The listing builds one solid part. Answer for the finished solid, in the listing's coordinates (mm). Round coordinates to 2 decimals unless told otherwise and drop trailing zeros. Order: outer loops, then holes, each group sorted by start corner. A loop starts at its lowest first (then second) coordinate and runs counter-clockwise, first axis right, second up. Notation, with made-up numbers: (-13, 54.5) -> (27, 54.5) arc R20 ccw to (27, 71.5) -> close; hole circle Ø10 at (50.5, -19). An arc over 180 degrees is marked (long way). Answer in a Markdown table with one row per item. Add a question column.
```python
from build123d import *

# Parameters (mm, degrees)
F3_START      = 698.5
F2_W          = 2438.4
F2_H          = 457.2
F2_R          = 38.1
F3_DEPTH      = 38.1
F4_DEPTH      = 736.6
F5_R          = 38.1
F6_DEPTH      = 228.6
F6_DEPTH_BACK = 228.6
F7_R          = 25.4
F8_SIZE       = 2.54


# Not quite as in the source:
# - a variable given as a bare number and used for a length is read in inches; the dataset says mm whatever the document's units were


with BuildPart() as f3:
    # F2 (on Top) → F3 (new body)
    with BuildSketch(Plane.XY.offset(F3_START)):
        Rectangle(F2_W, F2_H)
        with Locations((-914.4, 0)):
            Circle(F2_R, mode=Mode.SUBTRACT)
        with Locations((914.4, 0)):
            Circle(F2_R, mode=Mode.SUBTRACT)
        with Locations((-914.4, 0)):
            Circle(F2_R)
        with Locations((914.4, 0)):
            Circle(F2_R)
    extrude(amount=F3_DEPTH)

    # F2 (on Top) → F4 (join)
    with BuildSketch(Plane.XY):
        with Locations((-914.4, 0)):
            Circle(F2_R)
        with Locations((914.4, 0)):
            Circle(F2_R)
    extrude(amount=F4_DEPTH)

    # F5 (on Front) → F6 (join, two sides)
    with BuildSketch(Plane.XZ) as f6_sk:
        with Locations((-914.4, 0)):
            Circle(F5_R)
        with Locations((914.4, 0)):
            Circle(F5_R)
    extrude(amount=F6_DEPTH)
    extrude(f6_sk.sketch, amount=-F6_DEPTH_BACK)

    # F7
    f7_edges = [f3.edges().sort_by_distance(p)[0] for p in [
        (1219.2, -228.6, 717.55),
        (1219.2, 228.6, 717.55),
        (-1219.2, -228.6, 717.55),
        (-1219.2, 228.6, 717.55),
    ]]
    fillet(f7_edges, radius=F7_R)

    # F8
    f8_edges = [f3.edges().sort_by_distance(p)[0] for p in [
        (-1219.2, 0, 736.6),
        (-1211.760512, 221.160512, 736.6),
        (0, 228.6, 736.6),
        (-1211.760512, -221.160512, 736.6),
        (0, -228.6, 736.6),
        (1219.2, 0, 736.6),
        (1211.760512, 221.160512, 736.6),
        (1211.760512, -221.160512, 736.6),
    ]]
    chamfer(f8_edges, length=F8_SIZE)


solid = f3.part
```
Item 1: The part is cut by section C-C, the plane x = -914.4. Give the vertices of the cut face in (y, z), and give its area (3 significant figures).
Item 2: The part is cut by section D-D, the plane x = 425. Give the vertices of the cut face in (y, z).
Item 3: The part is cut by section B-B, the plane z = 433.5. Give the vertices of the cut face in (x, y).
Item 4: Find the intervals of material crossed by probe 1 along Z at (x, y) = (-232, -168.5); probe 2 along Z at (x, y) = (-920.5, 96.5); probe 3 along Z at (x, y) = (929, -77), in increasing order. Write a range as [from, to].
Item 5: The part is cut by section A-A, the plane y = 153. Give the vertices of the cut face in (x, z), and give its area (3 significant figures).
Item 6: For a pull along X with two mould halves and no side action, classify faces 1 (the face through (949.595, -14.593, 344.36)), 2 (the face through (-915, -228.6, 1)), 3 (the face through (-879.205, -14.593, 344.36)) as released by +X, released by -X, zero draft, split by the parting line, or undercut.
Item 7: A flat-ended cylindrical pin translates along its axis: P1, Ø2, axis at x = -730, y = -18.5, coming from the -Z side. Find the tip coordinate at first contact, or state that the pin passes through.
Resolved:
| question | item | result |
|---|---|---|
| 1 | outline | (-228.6, -38.1) -> (228.6, -38.1) -> (228.6, 38.1) -> (38.1, 38.1) -> (38.1, 698.5) -> (228.6, 698.5) -> (228.6, 734.06) -> (226.06, 736.6) -> (-226.06, 736.6) -> (-228.6, 734.06) -> (-228.6, 698.5) -> (-38.1, 698.5) -> (-38.1, 38.1) -> (-228.6, 38.1) -> close |
| 1 | area | 103,000 mm2 |
| 2 | outline | (-228.6, 698.5) -> (228.6, 698.5) -> (228.6, 734.06) -> (226.06, 736.6) -> (-226.06, 736.6) -> (-228.6, 734.06) -> close |
| 3 | outline | circle Ø76.2 at (-914.4, 0); circle Ø76.2 at (914.4, 0) |
| 4 | probe 1 | [698.5, 736.6] |
| 4 | probe 2 | [-37.61, 37.61], [698.5, 736.6] |
| 4 | probe 3 | [-35.19, 35.19], [698.5, 736.6] |
| 5 | outline | (-1219.2, 698.5) -> (1219.2, 698.5) -> (1219.2, 734.06) -> (1216.66, 736.6) -> (-1216.66, 736.6) -> (-1219.2, 734.06) -> close; circle Ø76.2 at (-914.4, 0); circle Ø76.2 at (914.4, 0) |
| 5 | area | 102,000 mm2 |
| 6 | face 1 | undercut |
| 6 | face 2 | zero draft |
| 6 | face 3 | undercut |
| 7 | P1 | z = 698.5 |
